```python
from build123d import *

# Parameters (mm, degrees)
F1_DEPTH = 18


# Not quite as in the source:
# - ends of sketch curves that miss each other by under 0.0002 mm in the source are joined


with BuildPart() as f1:
    # F0 (on Front) → F1 (new body)
    with BuildSketch(Plane.XZ):
        with BuildLine():
            ThreePointArc((-111.5625776076, -719.3076212806), (-111.5625776076, -713.6507670312), (-105.9057233581, -713.6507670312))
            Line((-105.9057233581, -713.6507670312), (-105.2886944829, -714.1507671559))
            Line((-105.2886944829, -714.1507671559), (-41.9563794829, -714.1507671559))
            Line((-41.9563794829, -714.1507671559), (-41.4683634829, -713.6507671559))
            ThreePointArc((-41.4683634829, -713.6507671559), (-35.8115093581, -713.6507670312), (-35.8115093581, -719.3076212806))
            Line((-35.8115093581, -719.3076212806), (-35.8094664829, -742.1509261559))
            ThreePointArc((-35.8094664829, -742.1509261559), (-35.2236167578, -743.5650240029), (-33.8094664829, -744.1507471559))
            Line((-33.8094664829, -744.1507471559), (18.4384905171, -744.1507471559))
            ThreePointArc((18.4384905171, -744.1507471559), (19.8527040795, -743.5649607183), (20.4384905171, -742.1507471559))
            Line((20.4384905171, -742.1507471559), (20.4384905171, -733.6507671559))
            ThreePointArc((20.4384905171, -733.6507671559), (19.8527040795, -732.2365535935), (18.4384905171, -731.6507671559))
            Line((18.4384905171, -731.6507671559), (4.0953445171, -731.6507671559))
            ThreePointArc((4.0953445171, -731.6507671559), (-1.5615098576, -731.6507670306), (-1.5615091076, -725.9939125312))
            Line((-1.5615091076, -725.9939125312), (-1.5615094829, -719.3076211559))
            ThreePointArc((-1.5615094829, -719.3076211559), (-1.5615096076, -713.6507670312), (4.0953446419, -713.6507670312))
            Line((4.0953446419, -713.6507670312), (5.0690155171, -714.6507671559))
            Line((5.0690155171, -714.6507671559), (20.4374225171, -714.6507671559))
            ThreePointArc((20.4374225171, -714.6507671559), (21.1445292983, -714.3578739371), (21.4374225171, -713.6507671559))
            Line((21.4374225171, -713.6507671559), (21.4374225171, 749.3492328441))
            ThreePointArc((21.4374225171, 749.3492328441), (21.1445292983, 750.0563396253), (20.4374225171, 750.3492328441))
            Line((20.4374225171, 750.3492328441), (5.1226495171, 750.3492328441))
            Line((5.1226495171, 750.3492328441), (4.0953445171, 749.3492328441))
            ThreePointArc((4.0953445171, 749.3492328441), (-1.5615098576, 749.3492329694), (-1.5615091076, 755.0060874688))
            Line((-1.5615091076, 755.0060874688), (-1.5615094829, 761.6923788441))
            ThreePointArc((-1.5615094829, 761.6923788441), (-1.5615096076, 767.3492329688), (4.0953446419, 767.3492329688))
            Line((4.0953446419, 767.3492329688), (18.4384905171, 767.3492328441))
            ThreePointArc((18.4384905171, 767.3492328441), (19.8527040795, 767.9350192817), (20.4384905171, 769.3492328441))
            Line((20.4384905171, 769.3492328441), (20.4384905171, 777.8492138441))
            ThreePointArc((20.4384905171, 777.8492138441), (19.8527040795, 779.2634274065), (18.4384905171, 779.8492138441))
            Line((18.4384905171, 779.8492138441), (-33.8094664829, 779.8492138441))
            ThreePointArc((-33.8094664829, 779.8492138441), (-35.2236171114, 779.2634903376), (-35.809466475, 777.8493918441))
            Line((-35.809466475, 777.8493918441), (-35.8115094829, 755.0060878441))
            ThreePointArc((-35.8115094829, 755.0060878441), (-35.8115091081, 749.3492329694), (-41.4683636076, 749.3492327194))
            Line((-41.4683636076, 749.3492327194), (-41.9683634829, 749.8492328441))
            Line((-41.9683634829, 749.8492328441), (-105.2468454829, 749.8492328441))
            Line((-105.2468454829, 749.8492328441), (-105.9057234829, 749.3492328441))
            ThreePointArc((-105.9057234829, 749.3492328441), (-111.5625778576, 749.3492329694), (-111.5625771076, 755.0060874688))
            Line((-111.5625771076, 755.0060874688), (-111.5625774829, 761.6923788441))
            ThreePointArc((-111.5625774829, 761.6923788441), (-111.5625776076, 767.3492329688), (-105.9057233581, 767.3492329688))
            Line((-105.9057233581, 767.3492329688), (-91.5625774829, 767.3492328441))
            ThreePointArc((-91.5625774829, 767.3492328441), (-90.1483639205, 767.9350192817), (-89.5625774829, 769.3492328441))
            Line((-89.5625774829, 769.3492328441), (-89.5625774829, 777.8492138441))
            ThreePointArc((-89.5625774829, 777.8492138441), (-90.1483639205, 779.2634274065), (-91.5625774829, 779.8492138441))
            Line((-91.5625774829, 779.8492138441), (-143.8105344829, 779.8492138441))
            ThreePointArc((-143.8105344829, 779.8492138441), (-145.2246851114, 779.2634903376), (-145.810534475, 777.8493918441))
            Line((-145.810534475, 777.8493918441), (-145.8125774829, 755.0060878441))
            ThreePointArc((-145.8125774829, 755.0060878441), (-145.8125771081, 749.3492329694), (-151.4694316076, 749.3492327194))
            Line((-151.4694316076, 749.3492327194), (-184.5625764829, 749.3492328441))
            ThreePointArc((-184.5625764829, 749.3492328441), (-185.9767900453, 748.7634464065), (-186.5625764829, 747.3492328441))
            Line((-186.5625764829, 747.3492328441), (-186.5625764829, -711.6507671559))
            ThreePointArc((-186.5625764829, -711.6507671559), (-185.9767900453, -713.0649807183), (-184.5625764829, -713.6507671559))
            Line((-184.5625764829, -713.6507671559), (-151.4694314829, -713.6507671559))
            ThreePointArc((-151.4694314829, -713.6507671559), (-145.8125773581, -713.6507670312), (-145.8125773581, -719.3076212806))
            Line((-145.8125773581, -719.3076212806), (-145.8105344829, -742.1509261559))
            ThreePointArc((-145.8105344829, -742.1509261559), (-145.2246847578, -743.5650240029), (-143.8105344829, -744.1507471559))
            Line((-143.8105344829, -744.1507471559), (-91.5625774829, -744.1507471559))
            ThreePointArc((-91.5625774829, -744.1507471559), (-90.1483639205, -743.5649607183), (-89.5625774829, -742.1507471559))
            Line((-89.5625774829, -742.1507471559), (-89.5625774829, -733.6507671559))
            ThreePointArc((-89.5625774829, -733.6507671559), (-90.1483639205, -732.2365535935), (-91.5625774829, -731.6507671559))
            Line((-91.5625774829, -731.6507671559), (-105.9057234829, -731.6507671559))
            ThreePointArc((-105.9057234829, -731.6507671559), (-111.5625778576, -731.6507670306), (-111.5625771076, -725.9939125312))
            Line((-111.5625771076, -725.9939125312), (-111.5625776076, -719.3076212806))
        make_face()
        with BuildLine():
            ThreePointArc((-82.3041508581, -276.4939125312), (-82.3041501081, -282.1507670306), (-87.9610046076, -282.1507672806))
            Line((-87.9610046076, -282.1507672806), (-152.4757234829, -282.1507671559))
            ThreePointArc((-152.4757234829, -282.1507671559), (-158.1325778576, -282.1507670306), (-158.1325771076, -276.4939125312))
            Line((-158.1325771076, -276.4939125312), (-158.1325774829, -269.8076211559))
            ThreePointArc((-158.1325774829, -269.8076211559), (-158.1325776076, -264.1507670312), (-152.4757233581, -264.1507670312))
            Line((-152.4757233581, -264.1507670312), (-87.9610044829, -264.1507671559))
            ThreePointArc((-87.9610044829, -264.1507671559), (-82.3041503581, -264.1507670312), (-82.3041503581, -269.8076212806))
            Line((-82.3041503581, -269.8076212806), (-82.3041508581, -276.4939125312))
        make_face(mode=Mode.SUBTRACT)
        with BuildLine():
            Line((-163.4866634829, -18.1507671559), (-163.4866634829, 53.8492328441))
            ThreePointArc((-163.4866634829, 53.8492328441), (-162.3150906076, 56.6776599688), (-159.4866634829, 57.8492328441))
            Line((-159.4866634829, 57.8492328441), (-87.4866634829, 57.8492328441))
            ThreePointArc((-87.4866634829, 57.8492328441), (-84.6582363581, 56.6776599688), (-83.4866634829, 53.8492328441))
            Line((-83.4866634829, 53.8492328441), (-83.4866634829, -18.1507671559))
            ThreePointArc((-83.4866634829, -18.1507671559), (-84.6582363581, -20.9791942806), (-87.4866634829, -22.1507671559))
            Line((-87.4866634829, -22.1507671559), (-159.4866634829, -22.1507671559))
            ThreePointArc((-159.4866634829, -22.1507671559), (-162.3150906076, -20.9791942806), (-163.4866634829, -18.1507671559))
        make_face(mode=Mode.SUBTRACT)
        with BuildLine():
            Line((-82.3041504829, 312.1923788441), (-82.3041504829, 305.5060878441))
            ThreePointArc((-82.3041504829, 305.5060878441), (-82.3041503581, 299.8492327194), (-87.9610046076, 299.8492327194))
            Line((-87.9610046076, 299.8492327194), (-152.4757234829, 299.8492328441))
            ThreePointArc((-152.4757234829, 299.8492328441), (-158.1325778576, 299.8492329694), (-158.1325771076, 305.5060874688))
            Line((-158.1325771076, 305.5060874688), (-158.1325774829, 312.1923788441))
            ThreePointArc((-158.1325774829, 312.1923788441), (-158.1325776076, 317.8492329688), (-152.4757233581, 317.8492329688))
            Line((-152.4757233581, 317.8492329688), (-87.9610044829, 317.8492328441))
            ThreePointArc((-87.9610044829, 317.8492328441), (-82.3041503581, 317.8492329688), (-82.3041504829, 312.1923788441))
        make_face(mode=Mode.SUBTRACT)
    extrude(amount=-F1_DEPTH)


solid = f1.part
```
The listing builds one solid part. Answer for the finished solid, in the listing's coordinates (mm). Give positions to 0.01 mm unless a question says otherwise; leave off trailing zeros. Order: outer loops, then holes, each group sorted by start corner. A loop starts at its lowest first (then second) coordinate and runs counter-clockwise, first axis right, second up. Notation, with made-up numbers: (43, -31) -> (72, -31) arc R7 cw to (72, -26) -> close; hole circle Ø7 at (41.5, -16). An arc over 180 degrees is marked (long way). Answer as CSV lines item,"result". Start each with the question number.
Q1. A cutting plane is placed at A-A (x = -126). Determine the outline of the cut face in (y, z), then the cut area to 3 significant figures.
Q2. A cutting plane is placed at B-B (x = -55.5). Determine the outline of the cut face in (y, z).
Q3. Given pin 1 (12 mm diameter, centred on x = -90.5, z = -300, fed in from -Y); pin 2 (5.5 mm diameter, centred on y = 8, z = 770, fed in from -X); pin 3 (8 mm diameter, centred on x = -43, y = 16, fed in from -Z); pin 4 (4 mm diameter, centred on y = 10, z = 774, fed in from +X), each flat-ended and moving along its own axis, determine where each tip first touches the part or whether it passes through.
Q4. Find the intervals of material crossed by L1, parallel to Z at x = 5, y = 11.25; L2, parallel to Z at x = -138.5, y = 8.5; L3, parallel to Z at x = -102.5, y = 15.25, in increasing order.
Q5. A cutting plane is placed at C-C (y = 3.5). Count the separate pieces of the cut face and the enclosed holes in it, then the cut area to 3 significant figures.
Results found:
1,outline,"(0, -744.15) -> (18, -744.15) -> (18, -282.15) -> (0, -282.15) -> close; (0, -264.15) -> (18, -264.15) -> (18, -22.15) -> (0, -22.15) -> close; (0, 57.85) -> (18, 57.85) -> (18, 299.85) -> (0, 299.85) -> close; (0, 317.85) -> (18, 317.85) -> (18, 779.85) -> (0, 779.85) -> close"
1,area,"25,300 mm2"
2,outline,"(0, -714.15) -> (18, -714.15) -> (18, 749.85) -> (0, 749.85) -> close"
3,pin 1,"y = 0"
3,pin 2,"x = -145.81"
3,pin 3,"z = -714.15"
3,pin 4,"x = 20.44"
4,L1,"-744.15 to -731.65, -714.58 to 750.23, 767.35 to 779.85"
4,L2,"-744.15 to -282.15, -264.15 to -22.15, 57.85 to 299.85, 317.85 to 779.85"
4,L3,"-744.15 to -731.65, -714.15 to -282.15, -264.15 to -22.15, 57.85 to 299.85, 317.85 to 749.85, 767.35 to 779.85"
5,separate pieces,"1"
5,enclosed holes,"3"
5,area,"300,000 mm2"
